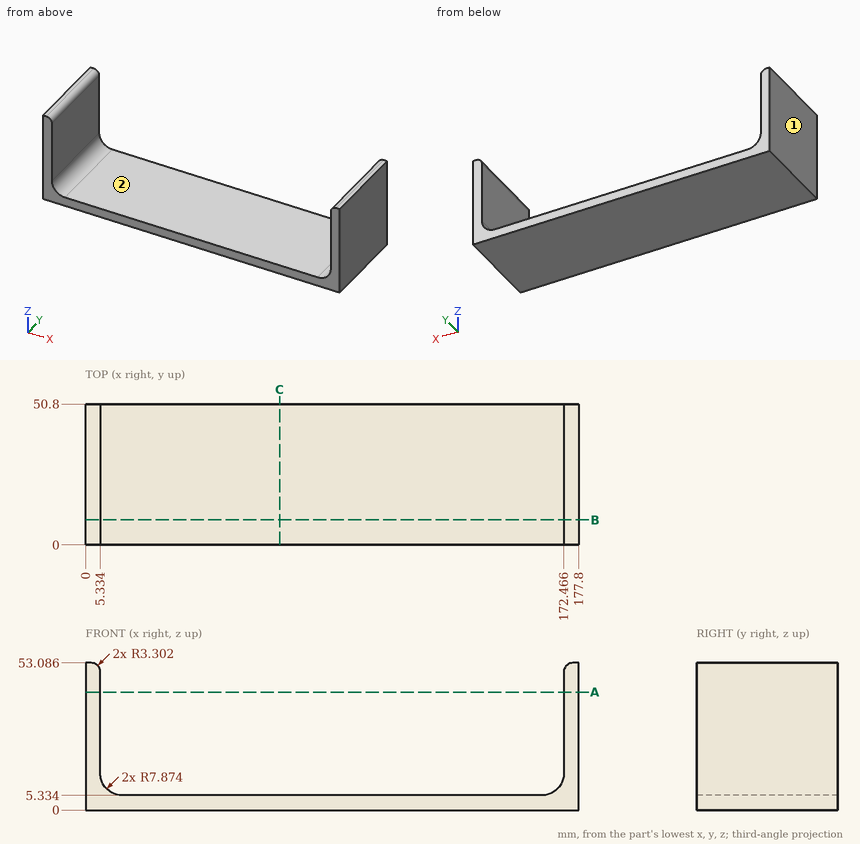
For this review, use the dimensioned drawing (mm, ordinates from the lowest corner) and the shaded views. A direction names the side the tool comes from. Round coordinates to 2 decimals unless told otherwise and drop trailing zeros. Write each loop counter-clockwise with the first axis right and the second up, starting at its lowest first coordinate (ties: lowest second). Pieces come first, ordered by that corner, then holes. Notation, with made-up numbers: (-6.75, -28.5) - (38.25, -28.5) arc R15 ccw to (38.25, -21.5) - close; hole circle Ø1 at (86.25, 72). An arc over 180 degrees is marked (long way). Use a Markdown table: item, result.
Q1. We need section B-B (y = 9). Give the boundary of the cut face in (x, z), plus the area to 3 significant figures.
Derived:
| item | result |
|---|---|
| outline | (0, 0) - (177.8, 0) - (177.8, 53.09) - (175.77, 53.09) arc R3.3 ccw to (172.47, 49.78) - (172.47, 13.21) arc R7.87 cw to (164.59, 5.33) - (13.21, 5.33) arc R7.87 cw to (5.33, 13.21) - (5.33, 49.78) arc R3.3 ccw to (2.03, 53.09) - (0, 53.09) - close |
| area | 1,480 mm2 |
Q2. Wall thickness on line 1 along X through (y, z) = (40, 37); line 2 along Z through (x, y) = (140.5, 7); line 3 along X through (y, z) = (5, 12): over which ranges is each line inside the solid? List them lowest first.
Derived:
| item | result |
|---|---|
| line 1 | x = 0 to 5.33, 172.47 to 177.8 |
| line 2 | z = 0 to 5.33 |
| line 3 | x = 0 to 5.43, 172.37 to 177.8 |
Q3. Machinability: for the marked faces 1 and 2, which of the approach directions +Z, -Z, +X, -X, +Y, -Y give a long, thin tool a straight path to every point of the face, cutting with its end or side? Answer none if there is none.
Derived:
| item | result |
|---|---|
| face 1 | +Z, -Z, -X, +Y, -Y |
| face 2 | +Z, +Y, -Y |
Q4. Clearance check with a flat-ended pin moving along its axis: pin 1 (8 mm diameter, centred on x = 20.5, y = 34.5, fed in from +Z). State where the tip first meets the part, or that it passes through.
Derived:
| item | result |
|---|---|
| pin 1 | stops at z = 5.33 |
Q5. We need section A-A (z = 42.5). Give the boundary of the cut face in (x, y), plus the area to 3 significant figures.
Derived:
| item | result |
|---|---|
| outline | (0, 0) - (5.33, 0) - (5.33, 50.8) - (0, 50.8) - close; (172.47, 0) - (177.8, 0) - (177.8, 50.8) - (172.47, 50.8) - close |
| area | 542 mm2 |
Q6. We need section C-C (x = 70). Give the boundary of the cut face in (y, z), plus the area to 3 significant figures.
Derived:
| item | result |
|---|---|
| outline | (0, 0) - (50.8, 0) - (50.8, 5.33) - (0, 5.33) - close |
| area | 271 mm2 |
